Geometry: final body of the model. Coordinates: model frame, mm. Give positions to 0.01 mm unless a question says otherwise; leave off trailing zeros. Order: outer loops, then holes, each group sorted by start corner. A loop starts at its lowest first (then second) coordinate and runs counter-clockwise, first axis right, second up. Notation, with made-up numbers: (-8, 42) - (20, 42) arc R23 cw to (20, 53) - close; hole circle Ø9 at (69, 81.25). An arc over 180 degrees is marked (long way). Put each result on its own line as item: value. Start each with the question number.
1. Section C-C on z = 21. Return the cut outline in (x, y).
2. First-contact query: P1, Ø1, axis at x = 1, y = -0.5, coming from the -Z side; P2, Ø0.6, axis at x = 1.5, z = 7.5, coming from the -Y side; P3, Ø2, axis at y = 0, z = 39, coming from the -X side. Flat tips, straight axial feed; report the tip coordinate or a pass-through.
3. Ray query, line 1 along X through (y, z) = (-0.3, 41); line 2 along Y through (x, z) = (0.5, 13.5); line 3 along Y through (x, z) = (0.6, 38.5). Return the intervals inside material, ascending. Write a range as from..to.
4. Section B-B on z = 7. Return the cut outline in (x, y), plus the area to 3 significant figures.
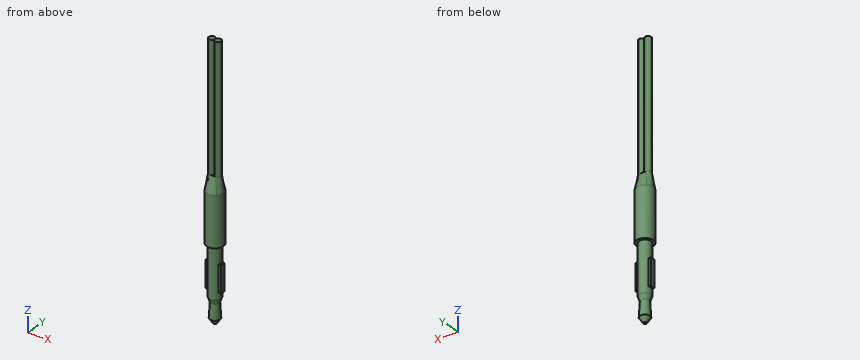
Autodesk Inventor part; units mm, degrees
ref_plane "Work Plane3" through (0, 0, 5) normal (0, 0, 1) x (1, 0, 0)
ref_plane "Work Plane4" through (0, 0, 28) normal (0, 0, 1) x (1, 0, 0)
ref_plane "Work Plane5" through (0, 0, 0) normal (1, 0, 0) x (0, 1, 0)
sketch "Sketch1" plane through (0, 0, 0) normal (0, 0, 1) x (1, 0, 0)
  circle A0 centre (0, 0) radius 0.3405
  dimension "d0" = 0.681
ref_plane "Work Plane1" through (0, 0, 1) normal (0, 0, 1) x (1, 0, 0)
sketch "Sketch2" plane through (0, 0, 1) normal (0, 0, 1) x (1, 0, 0)
  circle A0 centre (0, 0) radius 1.0215
  dimension "d2" = 2.043
ref_plane "Work Plane2" through (0, 0, 4) normal (0, 0, 1) x (1, 0, 0)
sketch "Sketch3" plane through (0, 0, 4) normal (0, 0, 1) x (1, 0, 0)
  circle A0 centre (0, 0) radius 0.8476
  dimension "d4" = 1.6951
ref_plane "Work Plane3" through (0, 0, 5) normal (0, 0, 1) x (1, 0, 0)
sketch "Sketch4" plane through (0, 0, 5) normal (0, 0, 1) x (1, 0, 0)
  circle A0 centre (0, 0) radius 1.1935
  dimension "d6" = 2.387
loft "Loft1" add profiles "Sketch4", "Sketch3"
loft "Loft2" add profiles "Sketch2" section 1 edges at (-0.8476, 0, 4)
loft "Loft3" add profiles "Sketch1" section 2 edges at (-1.0215, 0, 1)
sketch "Sketch5" plane through (0, 0, 5) normal (0, 0, 1) x (1, 0, 0)
  circle A0 centre (0, 0) radius 1.1906
  dimension "d35" = 2.3813
extrude "Extrusion1" add sketch "Sketch5" along normal blind 10
sketch "Sketch6" plane through (0, 0, 15) normal (0, 0, 1) x (1, 0, 0)
  circle A0 centre (0, 0) radius 1.7038
  dimension "d21" = 3.4076
extrude "Extrusion2" add sketch "Sketch6" along normal blind 10
ref_plane "Work Plane4" through (0, 0, 28) normal (0, 0, 1) x (1, 0, 0)
sketch "Sketch7" plane through (0, 0, 28) normal (0, 0, 1) x (1, 0, 0)
  arc A0 (-0.635, 0.635) -> (-0.635, -0.635) centre (-0.635, 0) ccw
  arc A1 (0.635, -0.635) -> (0.635, 0.635) centre (0.635, 0) ccw
  line L0 (-0.635, 0.635) -> (0.635, 0.635)
  line L1 (0.635, -0.635) -> (-0.635, -0.635)
loft "Loft4" add profiles "Sketch7" section 1 edges at (-1.7038, 0, 25)
sketch "Sketch8" plane through (0, 0, 28) normal (0, 0, 1) x (1, 0, 0)
  arc A0 (-0.635, 0.635) -> (-0.635, -0.635) centre (-0.635, 0) ccw
  circle A1 centre (-0.635, 0) radius 0.635
  arc A2 (0.635, -0.635) -> (0.635, 0.635) centre (0.635, 0) ccw
  circle A3 centre (0.635, 0) radius 0.635
  point P0 (0, 0)
extrude "Extrusion3" add sketch "Sketch8" along normal blind 25.4
ref_plane "Work Plane5" through (0, 0, 0) normal (1, 0, 0) x (0, 1, 0)
sketch "Sketch9" plane through (0, 0, 0) normal (1, 0, 0) x (0, 1, 0)
  line L0 (0.508, 11.571) -> (-0.508, 11.571)
  line L1 (-0.508, 11.571) -> (-0.508, 6.27)
  line L2 (-0.508, 6.27) -> (0.508, 6.27)
  line L3 (0.508, 6.27) -> (0.508, 11.571)
  line L4 (-1.7038, 15) -> (1.7038, 15)
  line L5 (-1.1935, 5) -> (1.1935, 5)
  point P0 (0, 0)
  dimension "d37" = 0.508
  dimension "d38" = 0.508
  dimension "d39" = 3.429
  dimension "d40" = 1.27
extrude "Extrusion4" add sketch "Sketch9" along normal mid plane 3.175
properties part number "Snap-Twist Idea M"
Resolved:
1. outline: circle Ø3.41 at (0, 0)
2. P1: z = 0.41
2. P2: y = -0.51
2. P3: x = -1.27
3. line 1: -1.19..-0.08, 0.08..1.19
3. line 2: -1.08..1.08
3. line 3: -0.63..0.63
4. outline: (-1.59, -0.51) - (-1.08, -0.51) arc R1.19 ccw to (1.08, -0.51) - (1.59, -0.51) - (1.59, 0.51) - (1.08, 0.51) arc R1.19 ccw to (-1.08, 0.51) - (-1.59, 0.51) - close
4. area: 5.34 mm^2
